The figure shows three views and two pictorial views of one solid part (mm, origin at its lowest corner). Answer the questions. A direction names the side the tool comes from. Round coordinates to 2 decimals unless told otherwise and drop trailing zeros. Order: outer loops, then holes, each group sorted by start corner. A loop starts at its lowest first (then second) coordinate and runs counter-clockwise, first axis right, second up. Notation, with made-up numbers: (-30.5, 4.5) - (-5.5, 4.5) arc R17 ccw to (-5.5, 31.5) - close; hole circle Ø6 at (64.25, -4.75). An arc over 180 degrees is marked (long way). Answer as a JSON object with one key per item and string values. Group by question number.
Q1. Consider line 1 (X direction, y = 5.5, z = 3.5). Determine where the line is inside the solid, lowest interval first.
Q2. A cutting plane is placed at B-B on y = 4. Determine the outline of the cut face in (x, z).
Q3. A cutting plane is placed at D-D on y = 0.75. Determine the outline of the cut face in (x, z), and give its area (3 significant figures).
Q4. A cutting plane is placed at C-C on x = 5.5. Determine the outline of the cut face in (y, z).
Q5. Given pin 1 Ø1.5 at (y, z) = (5.5, 12.5) entering from -X; pin 2 Ø1 at (x, y) = (27, 3.5) entering from -Z, each flat-ended and moving along its own axis, determine where each tip first touches the part or whether it passes through.
Q6. A tool of negligible diameter and unlimited length cuts with its end or side. For the marked faces 1 and 2, from which of +Z, -Z, +X, -X, +Y, -Y can it reach the whole face along a straight path? Write none if from no direction.
Q7. A cutting plane is placed at A-A on z = 7. Determine the outline of the cut face in (x, y).
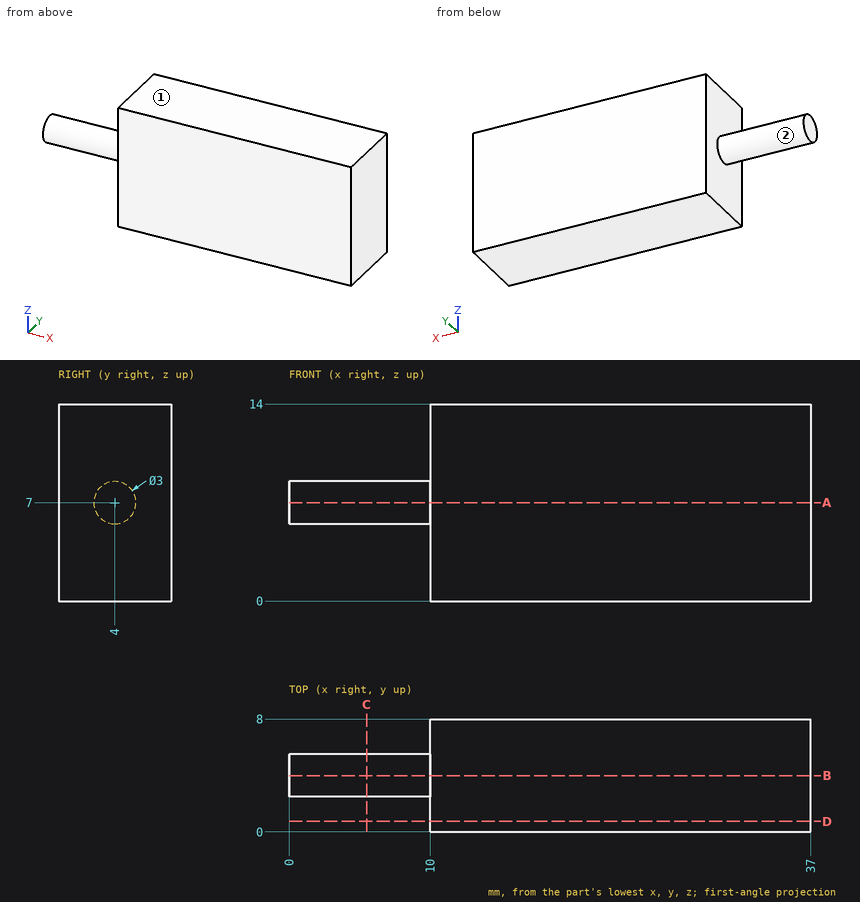
Result set:
{
 "1": {"line 1": "x = 10 to 37"},
 "2": {"outline": "(0, 5.5) - (10, 5.5) - (10, 0) - (37, 0) - (37, 14) - (10, 14) - (10, 8.5) - (0, 8.5) - close"},
 "3": {"outline": "(10, 0) - (37, 0) - (37, 14) - (10, 14) - close", "area": "378 mm²"},
 "4": {"outline": "circle Ø3 at (4, 7)"},
 "5": {"pin 1": "stops at x = 10", "pin 2": "stops at z = 0"},
 "6": {"face 1": "+Z, +X, -X, +Y, -Y", "face 2": "-X"},
 "7": {"outline": "(0, 2.5) - (10, 2.5) - (10, 0) - (37, 0) - (37, 8) - (10, 8) - (10, 5.5) - (0, 5.5) - close"}
}
